Work out the finished part from the listing and answer in its coordinate system (mm). Round coordinates to 2 decimals unless told otherwise and drop trailing zeros. Order: outer loops, then holes, each group sorted by start corner. A loop starts at its lowest first (then second) coordinate and runs counter-clockwise, first axis right, second up. Notation, with made-up numbers: (82, 51.25) -> (118, 51.25) arc R15 cw to (118, 60.25) -> close; hole circle Ø11 at (3, -28.75). An arc over 180 degrees is marked (long way). Use one line per item in the form item = value.
```python
from build123d import *

# Parameters (mm, degrees)
F0_W     = 350
F0_H     = 2180
F1_DEPTH = 9
F2_R     = 20
F3_DEPTH = 25


with BuildPart() as f1:
    # F0 (on Front) → F1 (new body, symmetric)
    with BuildSketch(Plane.XZ):
        Rectangle(F0_W, F0_H)
    extrude(amount=F1_DEPTH, both=True)

    # F2 (on face) → F3 (cut)
    with BuildSketch(Plane.XZ.offset(9)):
        with Locations((130, -885)):
            Circle(F2_R)
    extrude(amount=-F3_DEPTH, mode=Mode.SUBTRACT)


solid = f1.part
```
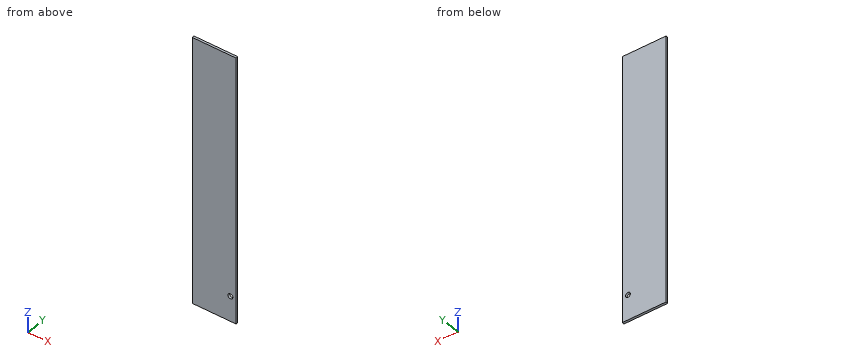
Item 1: The part is cut by section A-A, the plane x = 130. Give the vertices of the cut face in (y, z), and give its area (3 significant figures).
Findings:
outline = (-9, -1090) -> (9, -1090) -> (9, -905) -> (-9, -905) -> close; (-9, -865) -> (9, -865) -> (9, 1090) -> (-9, 1090) -> close
area = 38,500 mm^2
Item 2: Consider line 1 along Z through (x, y) = (130, -0.5); line 2 along Z through (x, y) = (136, 0). Determine where each line is inside the solid, lowest interval first.
Findings:
line_1 = -1090 to -905, -865 to 1090
line_2 = -1090 to -904.08, -865.92 to 1090
Item 3: The part is cut by section B-B, the plane z = -885. Give the vertices of the cut face in (x, y).
Findings:
outline = (-175, -9) -> (110, -9) -> (110, 9) -> (-175, 9) -> close; (150, -9) -> (175, -9) -> (175, 9) -> (150, 9) -> close
